from build123d import *

# Parameters (mm, degrees)
F2_R          = 1.75
F3_DEPTH      = 34.501
F4_R          = 1.6
F5_DEPTH      = 20.001
F5_DEPTH_BACK = 20.001
F6_R          = 1.6
F7_DEPTH      = 20.001
F7_DEPTH_BACK = 20.001
F8_C1_SIZE2   = 1.5
F8_C1_SIZE    = 1
F8_C2_SIZE2   = 1.5
F8_C2_SIZE    = 1


# Not quite as in the source:
# - two fillets or chamfers of one size are made in one step


with BuildPart() as f1:
    # F0 (on Front) → F1 (revolve)
    with BuildSketch(Plane.XZ):
        Polygon((0, 20), (0, 15), (34.5, 15), (34.5, 20), (21.5, 20), (20.3, 18.8), (15.2, 18.8), (14, 20), align=None)
    revolve(axis=Axis((0.4285710554, 0, 0), (1, 0, 0)))

    # F2 (on Right) → F3 (cut, through all)
    with BuildSketch(Plane.YZ):
        with Locations((14, 0)):
            Circle(F2_R)
        with Locations((0, 14)):
            Circle(F2_R)
        with Locations((-14, 0)):
            Circle(F2_R)
        with Locations((0, -14)):
            Circle(F2_R)
    extrude(amount=F3_DEPTH, mode=Mode.SUBTRACT)

    # F4 (on Top) → F5 (cut, two sides)
    with BuildSketch(Plane.XY) as f5_sk:
        with Locations((17.7, 0)):
            Circle(F4_R)
    extrude(amount=-F5_DEPTH, mode=Mode.SUBTRACT)
    extrude(f5_sk.sketch, amount=F5_DEPTH_BACK, mode=Mode.SUBTRACT)

    # F6 (on Front) → F7 (cut, two sides)
    with BuildSketch(Plane.XZ) as f7_sk:
        with Locations((17.8, 0)):
            Circle(F6_R)
    extrude(amount=-F7_DEPTH, mode=Mode.SUBTRACT)
    extrude(f7_sk.sketch, amount=F7_DEPTH_BACK, mode=Mode.SUBTRACT)

    # F8: chamfer of 1.5 x 1 on 2 edges, made by hand

    # F8_c1
    f8_c1_edges = [f1.edges().sort_by_distance(p)[0] for p in [
        (0, 0, -20),
    ]]
    f8_c1_side = f1.faces().sort_by_distance((0, 0, -19.98))[0]
    chamfer(f8_c1_edges, length=F8_C1_SIZE, length2=F8_C1_SIZE2, reference=f8_c1_side)

    # F8_c2
    f8_c2_edges = [f1.edges().sort_by_distance(p)[0] for p in [
        (34.5, 0, -20),
    ]]
    f8_c2_side = f1.faces().sort_by_distance((34.5, 0, -19.98))[0]
    chamfer(f8_c2_edges, length=F8_C2_SIZE, length2=F8_C2_SIZE2, reference=f8_c2_side)


solid = f1.part
Work out the finished part from the listing and answer in its coordinate system (mm). A direction names the side the tool comes from. Give positions to 0.01 mm unless a question says otherwise; leave off trailing zeros. Loops run counter-clockwise (first coordinate to the right, second up) from the corner with the lowest first, then second, coordinate; pieces in that order, holes last. Notation, with made-up numbers: (63.25, 72.5) -> (89.25, 72.5) arc R22 cw to (89.25, 109.5) -> close; hole circle Ø1 at (26, 21). An arc over 180 degrees is marked (long way). Use a Markdown table: item, result. Add a question column.
1. Section A-A on y = 0 is taken. Determine the outline of the cut face in (x, z), and give its area (3 significant figures).
2. Flat-ended cylindrical pins translate along their axes: pin 1 Ø5 at (x, z) = (17.5, -7.5) entering from -Y; pin 2 Ø4 at (y, z) = (6.5, -9.5) entering from +X; pin 3 Ø1 at (x, y) = (18, 11) entering from +Z; pin 4 Ø5 at (x, y) = (22, 15.5) entering from -Z. Find the tip coordinate at first contact, or state that the pin passes through.
3. Find the intervals of material crossed by probe 1 along X at (y, z) = (-16.1, 0); probe 2 along X at (y, z) = (0, -17.2); probe 3 along Z at (x, y) = (11, -10.5), in increasing order.
4. For faces 1 (the flat face through (0, 13, 8)), 2 (the cylindrical face through (17.49, -10.71, -10.5)), determine the directions among +Z, -Z, +X, -X, +Y, -Y from which every point of the face is accessible in a straight line to the end or side of a thin tool.
5. Section C-C on x = 3 is taken. Determine the outline of the cut face in (y, z).
6. Section B-B on z = 0 is taken. Determine the outline of the cut face in (x, y), and give its area (3 significant figures).
7. Determine the mould class of faces 3 (the cylindrical face through (8.43, 0.02, 15.75)), 4 (the cylindrical face through (16.43, -0.97, 16.83)), 5 (the cylindrical face through (17.49, 10.71, 10.5)), 6 (the cylindrical face through (17.714, 7.201, 17.366)) for opening direction Z: released by +Z, released by -Z, zero draft, split by the parting line, or undercut.
Results below:
| question | item | result |
|---|---|---|
| 1 | outline | (0, -19) -> (1.5, -20) -> (14, -20) -> (15.2, -18.8) -> (16.1, -18.8) -> (16.1, -15.75) -> (0, -15.75) -> close; (0, 15.75) -> (16.1, 15.75) -> (16.1, 18.8) -> (15.2, 18.8) -> (14, 20) -> (1.5, 20) -> (0, 19) -> close; (19.3, -18.8) -> (20.3, -18.8) -> (21.5, -20) -> (33, -20) -> (34.5, -19) -> (34.5, -15.75) -> (19.3, -15.75) -> close; (19.3, 15.75) -> (34.5, 15.75) -> (34.5, 19) -> (33, 20) -> (21.5, 20) -> (20.3, 18.8) -> (19.3, 18.8) -> close |
| 1 | area | 256 mm^2 |
| 2 | pin 1 | stops at y = -18.12 |
| 2 | pin 2 | passes through |
| 2 | pin 3 | stops at z = 15.59 |
| 2 | pin 4 | stops at z = -15.2 |
| 3 | probe 1 | x = 0 to 16.2, 19.4 to 34.5 |
| 3 | probe 2 | x = 0 to 16.1, 19.3 to 34.5 |
| 3 | probe 3 | z = -17.02 to -10.71, 10.71 to 17.02 |
| 4 | face 1 | +Z, -Z, -X, +Y, -Y |
| 4 | face 2 | +X, -X |
| 5 | outline | circle Ø40 at (0, 0); hole (-14.93, -1.48) arc R15 ccw to (-1.48, -14.93) arc R1.75 ccw to (1.48, -14.93) arc R15 ccw to (14.93, -1.48) arc R1.75 ccw to (14.93, 1.48) arc R15 ccw to (1.48, 14.93) arc R1.75 ccw to (-1.48, 14.93) arc R15 ccw to (-14.93, 1.48) arc R1.75 ccw to start |
| 6 | outline | (0, -19) -> (1.5, -20) -> (14, -20) -> (15.2, -18.8) -> (16.2, -18.8) -> (16.2, -15.75) -> (0, -15.75) -> close; (0, 15.75) -> (16.2, 15.75) -> (16.2, 18.8) -> (15.2, 18.8) -> (14, 20) -> (1.5, 20) -> (0, 19) -> close; (19.4, -18.8) -> (20.3, -18.8) -> (21.5, -20) -> (33, -20) -> (34.5, -19) -> (34.5, -15.75) -> (19.4, -15.75) -> close; (19.4, 15.75) -> (34.5, 15.75) -> (34.5, 19) -> (33, 20) -> (21.5, 20) -> (20.3, 18.8) -> (19.4, 18.8) -> close |
| 6 | area | 256 mm^2 |
| 7 | face 3 | undercut |
| 7 | face 4 | zero draft |
| 7 | face 5 | undercut |
| 7 | face 6 | split by the parting line |
